```python
from build123d import *
from OCP.BRepFilletAPI import BRepFilletAPI_MakeChamfer

# Parameters (mm, degrees)
AUFSATZ_LINEAR_AUSTRAGEN1_DEPTH    = 20
SKIZZE2_R                          = 1.65
SKIZZE2_R_2                        = 2.65
SCHNITT_LINEAR_AUSTRAGEN1_DEPTH    = 3
FASE1_SIZE                         = 5
FASE1_SIZE2                        = 8.660254038
FASE2_SIZE                         = 2
FASE2_SIZE2                        = 1.154700538
K_RPER_VERSCHIEBEN_KOPIEREN1_ANGLE = 90


with BuildPart() as part:
    # Skizze1 → Aufsatz-Linear austragen1 (new body)
    with BuildSketch(Plane.XY):
        Polygon((0, 0), (28.4, 0), (28.4, 2.5), (22.3, 2.5), (22.3, 3), (0, 3), align=None)
    extrude(amount=AUFSATZ_LINEAR_AUSTRAGEN1_DEPTH)

    # Skizze2 → Schnitt-Linear austragen1 (cut)
    with BuildSketch(Plane.XZ):
        with Locations(Location((4, 10, 0), (0, 0, 270))):
            Circle(SKIZZE2_R)
        with Locations(Location((18.3, 10, 0), (0, 0, 270))):
            Circle(SKIZZE2_R_2)
    extrude(amount=-SCHNITT_LINEAR_AUSTRAGEN1_DEPTH, mode=Mode.SUBTRACT)

    # Fase1
    fase1_edges = [part.edges().sort_by_distance(p)[0] for p in [
        (0, 1.5, 20),
        (0, 1.5, 0),
    ]]
    fase1_side = [part.faces().sort_by_distance(p)[0] for p in [
        (0, 1.5, 10),
    ]]
    chamfer(fase1_edges, length=FASE1_SIZE, length2=FASE1_SIZE2, reference=fase1_side[0])

    # Fase2: one chamfer whose edges measure the first distance from different faces: ONE call of the kernel's chamfer builder (chamfer() names one face for all edges)
    fase2_edges_1 = [part.edges().sort_by_distance(p)[0] for p in [
        (0, 3, 10),
    ]]
    fase2_side_1 = [part.faces().sort_by_distance(p)[0] for p in [
        (0, 1.5, 10),
    ]]
    fase2_edges_2 = [part.edges().sort_by_distance(p)[0] for p in [
        (4.330127019, 3, 17.5),
    ]]
    fase2_side_2 = [part.faces().sort_by_distance(p)[0] for p in [
        (4.330127019, 1.5, 17.5),
    ]]
    fase2_edges_3 = [part.edges().sort_by_distance(p)[0] for p in [
        (4.330127019, 3, 2.5),
    ]]
    fase2_side_3 = [part.faces().sort_by_distance(p)[0] for p in [
        (4.330127019, 1.5, 2.5),
    ]]
    fase2 = BRepFilletAPI_MakeChamfer(part.part.solid().wrapped)
    for e in fase2_edges_1:
        fase2.Add(FASE2_SIZE, FASE2_SIZE2, e.wrapped, fase2_side_1[0].wrapped)  # the first distance lies on this face
    for e in fase2_edges_2:
        fase2.Add(FASE2_SIZE, FASE2_SIZE2, e.wrapped, fase2_side_2[0].wrapped)  # the first distance lies on this face
    for e in fase2_edges_3:
        fase2.Add(FASE2_SIZE, FASE2_SIZE2, e.wrapped, fase2_side_3[0].wrapped)  # the first distance lies on this face
    add(Compound.cast(fase2.Shape()), mode=Mode.REPLACE)


with BuildPart() as part_1:
    # Körper-Verschieben/Kopieren1: moved
    add(part.part.rotate(Axis((0, 1.5, 10), (1, 0, 0)), K_RPER_VERSCHIEBEN_KOPIEREN1_ANGLE))


solid = part_1.part
```
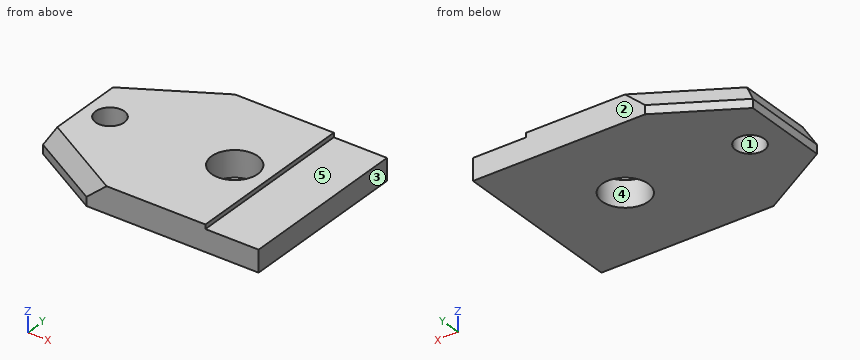
For this review, take the finished solid that the model builds, in its own axes (mm). Face numbers are marked on the shaded views. A direction names the side the tool comes from. Coordinates: 2 decimals unless noted, no trailing zeros. Loops run counter-clockwise (first coordinate to the right, second up) from the corner with the lowest first, then second, coordinate; pieces in that order, holes last.
1. Insertion check: P1, Ø3, axis at x = 24, y = -0.5, coming from the +Z side; P2, Ø4, axis at x = 18.3, y = 1.5, coming from the -Z side. Each pin has a flat end and moves straight along its axis. Give the tip position at first contact, or say it passes through.
2. For line 1 (X direction, y = 1.5, z = 10.55); line 2 (X direction, y = 1.5, z = 10.2); line 3 (Z direction, x = 27, y = 6.75), list the stretches that pass through material, from the lowest coordinate up.
3. Add section A-A, the plane x = 18.3. Give the boundary of the cut face in (y, z), then the cut area to 3 significant figures.
4. Add section D-D, the plane x = 4. Give the boundary of the cut face in (y, z), then the cut area to 3 significant figures.
5. Mouldability with a two-part tool opening along X and no side actions: class the marked faces 1, 2 and 3 as +X half, -X half, draft (parallel to the pull), parting line (faces both ways), or undercut.
6. Add section B-B, the plane y = 2. Give the boundary of the cut face in (x, z), then the cut area to 3 significant figures.
7. Add section C-C, the plane z = 9.2. Give the boundary of the cut face in (x, y).
8. For the marked faces 4 and 5, list the 3-axis set-ups (+Z, -Z, +X, -X, +Y, -Y) from which the entire face can be reached by the end or side of a thin tool; tool diameter is ignored.
Result:
1. P1: stops at z = 11
1. P2: passes through
2. line 1: x = 0.61 to 2.35, 5.65 to 15.65, 20.95 to 28.4
2. line 2: x = 0.4 to 2.35, 5.65 to 15.65, 20.95 to 28.4
2. line 3: z = 8.5 to 11
3. outline: (-8.5, 8.5) - (-1.15, 8.5) - (-1.15, 11.5) - (-8.5, 11.5) - close; (4.15, 8.5) - (11.5, 8.5) - (11.5, 11.5) - (4.15, 11.5) - close
3. area: 44.1 mm2
4. outline: (-5.81, 8.5) - (-0.15, 8.5) - (-0.15, 11.5) - (-4.48, 11.5) - (-5.81, 9.5) - close; (3.15, 8.5) - (8.81, 8.5) - (8.81, 9.5) - (7.48, 11.5) - (3.15, 11.5) - close
4. area: 31.3 mm2
5. face 1: undercut
5. face 2: draft
5. face 3: +X half
6. outline: (0, 8.5) - (2.43, 8.5) - (2.43, 11.5) - (1.15, 11.5) - (0, 9.5) - close; (5.57, 8.5) - (15.7, 8.5) - (15.7, 11.5) - (5.57, 11.5) - close; (20.9, 8.5) - (28.4, 8.5) - (28.4, 11) - (22.3, 11) - (22.3, 11.5) - (20.9, 11.5) - close
6. area: 55.9 mm2
7. outline: (0, -3.5) - (8.66, -8.5) - (28.4, -8.5) - (28.4, 11.5) - (8.66, 11.5) - (0, 6.5) - close; hole circle Ø3.3 at (4, 1.5); hole circle Ø5.3 at (18.3, 1.5)
8. face 4: +Z, -Z
8. face 5: +Z, +X, +Y, -Y
